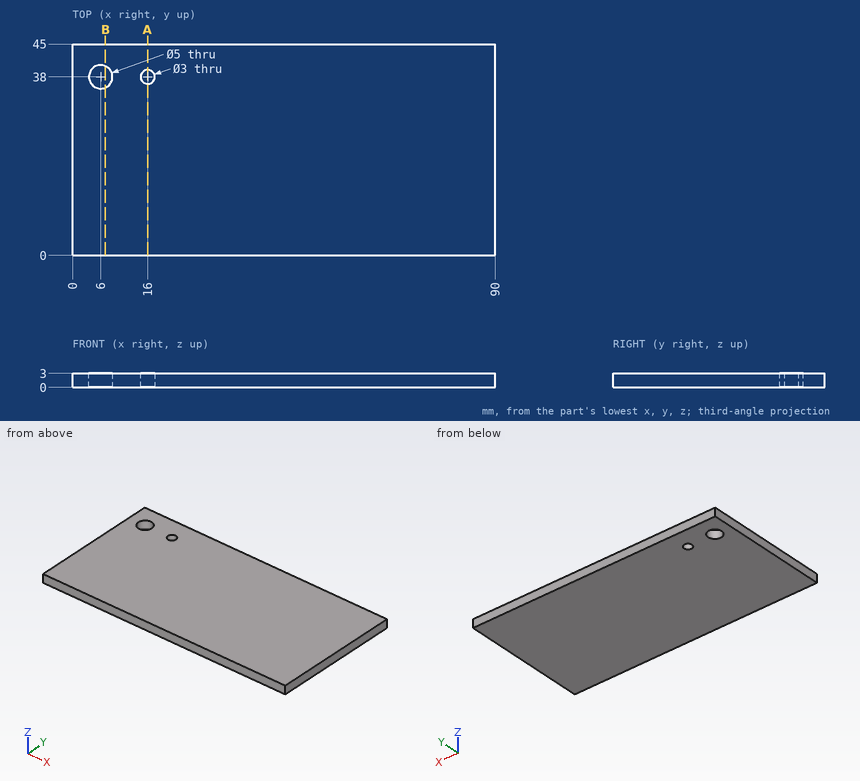
Part print with two shaded views. Sizes in mm from the minimum x, y, z corner. Round coordinates to 2 decimals unless told otherwise and drop trailing zeros. Loops run counter-clockwise (first coordinate to the right, second up) from the corner with the lowest first, then second, coordinate; pieces in that order, holes last. Notation, with made-up numbers: (7.5, -14.75) - (38.5, -14.75) arc R23 cw to (38.5, 9.25) - close; hole circle Ø1 at (-16.5, -30.5). An arc over 180 degrees is marked (long way). Answer as a JSON object with one key per item and string values.
Item 1: Band-saw the part on B-B on x = 7. List the corners of the cut face in (y, z), plus the area to 3 significant figures.
Output:
{"outline": "(0, 0) - (35.71, 0) - (35.71, 3) - (0, 3) - close; (40.29, 0) - (45, 0) - (45, 3) - (40.29, 3) - close", "area": "121 mm2"}
Item 2: Pin check, flat tip, straight feed: pin 1 (6 mm diameter, centred on x = 6, y = 38, fed in from -Z). Stop position of the tip, or through.
Output:
{"pin 1": "z = 0"}
Item 3: Wall check: L1, parallel to Y at x = 6, z = 2.3. Give the ranges that are in metal, low to high.
Output:
{"L1": "0 to 35.5, 40.5 to 45"}
Item 4: Band-saw the part on A-A on x = 16. List the corners of the cut face in (y, z).
Output:
{"outline": "(0, 0) - (36.5, 0) - (36.5, 3) - (0, 3) - close; (39.5, 0) - (45, 0) - (45, 3) - (39.5, 3) - close"}
